Work out the finished part from the listing and answer in its coordinate system (mm). A direction names the side the tool comes from. Round coordinates to 2 decimals unless told otherwise and drop trailing zeros. Loops run counter-clockwise (first coordinate to the right, second up) from the corner with the lowest first, then second, coordinate; pieces in that order, holes last.
```python
from build123d import *

# Parameters (mm, degrees)
SKETCH_1_W          = 240
SKETCH_1_H          = 90
EXTRUDE_1_DEPTH     = 4
SKETCH_2_W          = 170
SKETCH_2_H          = 90
EXTRUDE_2_DEPTH     = 6
SKETCH_3_R          = 3
CUT_EXTRUDE_1_DEPTH = 257.390327431
SKETCH_4_R          = 2.5
CUT_EXTRUDE_5_DEPTH = 257.515106768


with BuildPart() as part:
    # 草图1 → 凸台-拉伸1 (new body)
    with BuildSketch(Plane(origin=(0, 0, 0), x_dir=(1, 0, 0), z_dir=(0, 1, 0))):
        with Locations((120, -45)):
            Rectangle(SKETCH_1_W, SKETCH_1_H)
    extrude(amount=EXTRUDE_1_DEPTH)

    # 草图2 → 凸台-拉伸2 (add)
    with BuildSketch(Plane(origin=(0, 4, 0), x_dir=(1, 0, 0), z_dir=(0, 1, 0))):
        with Locations((120, -45)):
            Rectangle(SKETCH_2_W, SKETCH_2_H)
    extrude(amount=EXTRUDE_2_DEPTH)

    # 草图3 → 切除-拉伸1 (cut, through all)
    with BuildSketch(Plane(origin=(0, 4, 0), x_dir=(1, 0, 0), z_dir=(0, 1, 0))):
        with Locations(Location((17.5, -15, 0), (0, 0, 270))):
            Circle(SKETCH_3_R)
        with Locations(Location((17.5, -30, 0), (0, 0, 270))):
            Circle(SKETCH_3_R)
        with Locations(Location((17.5, -45, 0), (0, 0, 270))):
            Circle(SKETCH_3_R)
        with Locations(Location((17.5, -60, 0), (0, 0, 270))):
            Circle(SKETCH_3_R)
        with Locations(Location((17.5, -75, 0), (0, 0, 270))):
            Circle(SKETCH_3_R)
        with Locations(Location((222.5, -75, 0), (0, 0, 90))):
            Circle(SKETCH_3_R)
        with Locations(Location((222.5, -60, 0), (0, 0, 90))):
            Circle(SKETCH_3_R)
        with Locations(Location((222.5, -45, 0), (0, 0, 90))):
            Circle(SKETCH_3_R)
        with Locations(Location((222.5, -30, 0), (0, 0, 90))):
            Circle(SKETCH_3_R)
        with Locations(Location((222.5, -15, 0), (0, 0, 90))):
            Circle(SKETCH_3_R)
    extrude(amount=-CUT_EXTRUDE_1_DEPTH, mode=Mode.SUBTRACT)

    # 草图4 → 切除-拉伸5 (cut, through all)
    with BuildSketch(Plane.XZ):
        with Locations(Location((85, 81, 0), (0, 0, 270))):
            Circle(SKETCH_4_R)
        with Locations(Location((155, 81, 0), (0, 0, 270))):
            Circle(SKETCH_4_R)
        with Locations(Location((85, 31, 0), (0, 0, 270))):
            Circle(SKETCH_4_R)
        with Locations(Location((155, 31, 0), (0, 0, 270))):
            Circle(SKETCH_4_R)
        with Locations(Location((85, 51, 0), (0, 0, 270))):
            Circle(SKETCH_4_R)
        with Locations(Location((155, 51, 0), (0, 0, 270))):
            Circle(SKETCH_4_R)
    extrude(amount=-CUT_EXTRUDE_5_DEPTH, mode=Mode.SUBTRACT)


solid = part.part
```
1. Find section D-D (x = 31.5). Write down the section's boundary in (y, z), then the cut area to 3 significant figures.
Answer key:
outline: (0, 0) - (4, 0) - (4, 90) - (0, 90) - close
area: 360 mm2
2. Find section A-A (z = 51). Write down the section's boundary in (x, y), then the cut area to 3 significant figures.
Answer key:
outline: (0, 0) - (82.5, 0) - (82.5, 10) - (35, 10) - (35, 4) - (0, 4) - close; (87.5, 0) - (152.5, 0) - (152.5, 10) - (87.5, 10) - close; (157.5, 0) - (240, 0) - (240, 4) - (205, 4) - (205, 10) - (157.5, 10) - close
area: 1,880 mm2
3. Consider probe 1 along X at (y, z) = (1.95, 45); probe 2 along Z at (x, y) = (155, 2); probe 3 along X at (y, z) = (8, 81). Determine where each line is inside the solid, lowest interval first.
Answer key:
probe 1: x = 0 to 14.5, 20.5 to 219.5, 225.5 to 240
probe 2: z = 0 to 28.5, 33.5 to 48.5, 53.5 to 78.5, 83.5 to 90
probe 3: x = 35 to 82.5, 87.5 to 152.5, 157.5 to 205
4. Determine the mould class of faces 1 (the face through (219.526, 2.028, 30.391)), 2 (the face through (118, 5, 90)), 3 (the face through (15.7, 2, 72.6)), 4 (the face through (35, 7, 46)) for opening direction Z: +Z half, -Z half, draft (parallel to the pull), parting line (faces both ways), or undercut.
Answer key:
face 1: undercut
face 2: +Z half
face 3: undercut
face 4: draft
5. Find section C-C (z = 21.5). Write down the section's boundary in (x, y).
Answer key:
outline: (0, 0) - (240, 0) - (240, 4) - (205, 4) - (205, 10) - (35, 10) - (35, 4) - (0, 4) - close
6. Which of the six approach directions +Z, -Z, +X, -X, +Y, -Y give full straight-line access (tool end or side, diameter ignored) to faces 5 (the face through (13, 4, 44)), 6 (the face through (17.6, 2, 57)), 7 (the face through (226, 4, 44))?
Answer key:
face 5: +Z, -Z, -X, +Y
face 6: +Y, -Y
face 7: +Z, -Z, +X, +Y
7. Find section B-B (y = 6). Write down the section's boundary in (x, z).
Answer key:
outline: (35, 0) - (205, 0) - (205, 90) - (35, 90) - close; hole circle Ø5 at (85, 31); hole circle Ø5 at (85, 51); hole circle Ø5 at (85, 81); hole circle Ø5 at (155, 31); hole circle Ø5 at (155, 51); hole circle Ø5 at (155, 81)
8. Given pin 1 (3.5 mm diameter, centred on x = 17.5, z = 15, fed in from +Y); pin 2 (5 mm diameter, centred on y = 7.5, z = 64.5, fed in from +X); pin 3 (7 mm diameter, centred on x = 17.5, z = 30, fed in from -Y); pin 4 (17.5 mm diameter, centred on x = 228, z = 41.5, fed in from +Y), each flat-ended and moving along its own axis, determine where each tip first touches the part or whether it passes through.
Answer key:
pin 1: passes through
pin 2: stops at x = 205
pin 3: stops at y = 0
pin 4: stops at y = 4
